Build history of the part. All positions in model axes, mm. A direction names the side the tool comes from. Round coordinates to 2 decimals unless told otherwise and drop trailing zeros. Write each loop counter-clockwise with the first axis right and the second up, starting at its lowest first coordinate (ties: lowest second). Pieces come first, ordered by that corner, then holes.
Item 1: Wall check: probe 1 along Y at (x, z) = (-35, 1.25); probe 2 along Z at (x, y) = (30, 0.5); probe 3 along X at (y, z) = (0.5, -0.5). Give the ranges that are in metal, low to high.
Item 2: Band-saw the part on C-C, the plane x = -14.5. Write the cut outline in (y, z).
Item 3: 3-axis set-ups, long thin cutter, end or side, ignore diameter. For faces 4 (the flat face through (-1, -5, 1)), 5 (the flat face through (-1, 5, 1)), 6 (the flat face through (0.385, -5.708, -26.701)), 7 (the flat face through (27.5, -3, -23)): which of +Z, -Z, +X, -X, +Y, -Y reach the whole face in a straight line?
Item 4: Band-saw the part on B-B, the plane y = -3. Write the cut outline in (x, z).
Item 5: Drop flat-ended pins along their axis: pin 1 Ø1.5 at (y, z) = (-6, -26) entering from +X; pin 2 Ø12 at (x, z) = (20.5, -40.5) entering from +Y; pin 3 Ø3.5 at (x, y) = (35, 0) entering from +Z; pin 4 Ø1.5 at (x, z) = (-7, 1.5) entering from -Y. Give the stop position or say it passes through.
Item 6: Band-saw the part on A-A, the plane x = 35. Write the cut outline in (y, z), then the cut area to 3 significant figures.
Item 7: Mould opens along Y. For faces 1 (the flat face through (-27.5, -3, -23)), 2 (the cylindrical face through (33.4, 0.07, 1.48)), 3 (the flat face through (-38, 4, 1)) say: +Y half, -Y half, draft (parallel to the pull), parting line (faces both ways), or undercut.
```python
from build123d import *

# Parameters (mm, degrees)
SKETCH243_W     = 80
SKETCH243_H     = 10
SKETCH243_R     = 1.6
PAD126_DEPTH    = 3
CHAMFER087_SIZE = 3
PAD127_DEPTH    = 27.5
CHAMFER088_SIZE = 3
FILLET084_R     = 3


with BuildPart() as part:
    # Sketch243 → Pad126 (new body)
    with BuildSketch(Plane.XY):
        Rectangle(SKETCH243_W, SKETCH243_H)
        with Locations((35, 0)):
            Circle(SKETCH243_R, mode=Mode.SUBTRACT)
        with Locations((-35, 0)):
            Circle(SKETCH243_R, mode=Mode.SUBTRACT)
    extrude(amount=PAD126_DEPTH)

    # Chamfer087
    chamfer087_edges = [part.edges().sort_by_distance(p)[0] for p in [
        (40, -5, 1.5),
        (40, 5, 1.5),
        (-40, -5, 1.5),
        (-40, 5, 1.5),
    ]]
    chamfer(chamfer087_edges, length=CHAMFER087_SIZE)

    # Sketch244 → Pad127 (join, symmetric)
    with BuildSketch(Plane.YZ):
        Polygon((-1, 0), (2, 0), (-6.77287, -49.753418), (-9.682409, -49.240388), align=None)
    extrude(amount=PAD127_DEPTH, both=True)

    # Chamfer088
    chamfer088_edges = [part.edges().sort_by_distance(p)[0] for p in [
        (-27.5, -8.227639, -49.496903),
        (27.5, -8.227639, -49.496903),
    ]]
    chamfer(chamfer088_edges, length=CHAMFER088_SIZE)

    # Fillet084
    fillet084_edges = [part.edges().sort_by_distance(p)[0] for p in [
        (0, -1, 0),
        (0, 2, 0),
    ]]
    fillet(fillet084_edges, radius=FILLET084_R)


solid = part.part
```
Results:
1. probe 1: y = -5 to -1.6, 1.6 to 5
1. probe 2: z = 0 to 3
1. probe 3: x = -27.5 to 27.5
2. outline: (-9.68, -49.24) - (-6.77, -49.75) - (1.56, -2.48) arc R3 cw to (4.52, 0) - (5, 0) - (5, 3) - (-5, 3) - (-5, 0) - (-4.58, 0) arc R3 cw to (-1.62, -3.52) - close
3. face 4: +Z, +X, -X, -Y
3. face 5: +Z, -Z, +X, -X, +Y
3. face 6: +X, -X, -Y
3. face 7: -Z, +X, +Y, -Y
4. outline: (-39, 0) - (-27.5, 0) - (-27.5, -0.45) - (27.5, -0.45) - (27.5, 0) - (39, 0) - (39, 3) - (-39, 3) - close; (-27.5, -28.36) - (27.5, -28.36) - (27.5, -11.34) - (-27.5, -11.34) - close
5. pin 1: stops at x = 27.5
5. pin 2: stops at y = -4.08
5. pin 3: stops at z = 3
5. pin 4: stops at y = -5
6. outline: (-5, 0) - (-1.6, 0) - (-1.6, 3) - (-5, 3) - close; (1.6, 0) - (5, 0) - (5, 3) - (1.6, 3) - close
6. area: 20.4 mm2
7. face 1: draft
7. face 2: undercut
7. face 3: +Y half
